Design review of the part built by this model. Coordinates are the model's own, in mm. A direction names the side the tool comes from. Give positions to 0.01 mm unless a question says otherwise; leave off trailing zeros. Loops run counter-clockwise (first coordinate to the right, second up) from the corner with the lowest first, then second, coordinate; pieces in that order, holes last. Notation, with made-up numbers: (8, 37) - (20, 37) arc R22 cw to (20, 55) - close; hole circle Ø1 at (57, -2.75). An arc over 180 degrees is marked (long way). Write each question's results on one line, items separated by ' | '.
from build123d import *

# Parameters (mm, degrees)
SCHIZZO1_R                   = 17.5
ESTRUSIONE_ESTRUSIONE1_DEPTH = 50
TAGLIO_ESTRUSIONE1_REACH     = 145.634
SCHIZZO10_R                  = 16.3
SKETCH1_R                    = 16.3
SKETCH1_R_2                  = 14.8
BOSS_EXTRUDE3_DEPTH          = 15
SKETCH2_R                    = 2.2
BOSS_EXTRUDE4_DEPTH          = 5


# Read off the part's stored shape, not the designer's step: Rivoluzione1
with BuildPart() as part:
    # Schizzo1 → Estrusione-Estrusione1 (new body)
    with BuildSketch(Plane(origin=(0, 0, 0), x_dir=(1, 0, 0), z_dir=(0, 1, 0))):
        with Locations(Location((0, 0, 0), (0, 0, 270))):
            Circle(SCHIZZO1_R)
    extrude(amount=ESTRUSIONE_ESTRUSIONE1_DEPTH)

    # Rivoluzione1 outline → Rivoluzione1 (revolve)
    with BuildSketch(Plane.XY):
        with BuildLine():
            ThreePointArc((2.55, 139.999999998), (1.475612648, 141.087167398), (0, 141.485675179))
            Line((0, 141.485675179), (0, 138.8))
            Line((0, 138.8), (2, 138.8))
            add(Edge.make_bspline(
                [(2, 138.8), (16.3, 113.62789219), (16.3, 50)],
                knots=[0, 0, 0, 1, 1, 1], degree=2))
            Line((16.3, 50), (17.5, 50))
            add(Edge.make_bspline(
                [(17.5, 50), (17.5, 113.62789219), (2.55, 139.999999998)],
                knots=[0.022396988, 0.022396988, 0.022396988, 1.022396988, 1.022396988, 1.022396988], degree=2))
        make_face()
    revolve(axis=Axis((0, 0, 0), (0, 1, 0)))

    # Schizzo10 → Taglio-Estrusione1 (cut, up to next)
    with BuildSketch(Plane(origin=(0, 0, 0), x_dir=(1, 0, 0), z_dir=(0, 1, 0)), mode=Mode.PRIVATE) as taglio_estrusione1_sk1:
        with Locations(Location((0, 0, 0), (0, 0, 270))):
            Circle(SCHIZZO10_R)
    taglio_estrusione1_tool1 = extrude(taglio_estrusione1_sk1.sketch, amount=TAGLIO_ESTRUSIONE1_REACH, mode=Mode.PRIVATE) & part.part
    add(taglio_estrusione1_tool1.solids().sort_by_distance((0, 0, 0))[0], mode=Mode.SUBTRACT)

    # Sketch1 → Boss-Extrude3 (add)
    with BuildSketch(Plane.XZ):
        with Locations(Location((0, 0, 0), (0, 0, 270))):
            Circle(SKETCH1_R)
        with Locations(Location((0, 0, 0), (0, 0, 270))):
            Circle(SKETCH1_R_2, mode=Mode.SUBTRACT)
    extrude(amount=-BOSS_EXTRUDE3_DEPTH)

    # Sketch2 → Boss-Extrude4 (add)
    # profile 1 of 2: a face of its own
    with BuildSketch(Plane.XZ):
        with BuildLine():
            ThreePointArc((8.3, 4.3829214), (3.9170786, 0), (8.3, -4.3829214))
            Line((8.3, -4.3829214), (14.136123938, -4.3829214))
            ThreePointArc((14.136123938, -4.3829214), (14.8, 0), (14.136123938, 4.3829214))
            Line((14.136123938, 4.3829214), (8.3, 4.3829214))
        make_face()
        with Locations(Location((8.3, 0, 0), (0, 0, 270))):
            Circle(SKETCH2_R, mode=Mode.SUBTRACT)
    # profile 2 of 2: a face of its own
    with BuildSketch(Plane.XZ):
        with BuildLine():
            Line((-8.3, 4.3829214), (-14.136123938, 4.3829214))
            ThreePointArc((-14.136123938, 4.3829214), (-14.8, 0), (-14.136123938, -4.3829214))
            Line((-14.136123938, -4.3829214), (-8.3, -4.3829214))
            ThreePointArc((-8.3, -4.3829214), (-3.9170786, 0), (-8.3, 4.3829214))
        make_face()
        with Locations(Location((-8.3, 0, 0), (0, 0, 270))):
            Circle(SKETCH2_R, mode=Mode.SUBTRACT)
    extrude(amount=-BOSS_EXTRUDE4_DEPTH)


solid = part.part
(1) Draft analysis for pull direction Y (two halves, no side actions). For faces 1 (the flat face through (-11, 5, 0)), 2 (the cylindrical face through (-10.448, 2.465, 0.477)), 3 (the flat face through (4.1, 0, 0.2)), state which applies: pulls with the +Y half, pulls with the -Y half, needs draft (parallel to the pull), parting line crosses it, or undercut.
Answers below:
face 1: undercut | face 2: needs draft | face 3: pulls with the -Y half
(2) Insertion check: P1, Ø1, axis at y = 76.5, z = 11, coming from the +X side; P2, Ø2.5, axis at x = -7.5, z = 1.5, coming from the +Y side; P3, Ø4.5, axis at x = -0.5, z = -0.5, coming from the -Y side. Each pin has a flat end and moves straight along its axis. Give the tip position at first contact, or say it passes through.
Answers below:
P1: x = 13.06 | P2: y = 131.99 | P3: y = 137.04
(3) Take a section at A-A on y = 40. Give the boundary of the cut face in (x, z), plus the area to 3 significant figures.
Answers below:
outline: circle Ø35 at (0, 0); hole circle Ø32.6 at (0, 0) | area: 127 mm2
(4) Wall thickness on line 1 along X through (y, z) = (3, 0); line 2 along Z through (x, y) = (0, 30); line 3 along X through (y, z) = (8.25, 0): over which ranges is each line inside the solid? List them lowest first. Write a range as from..to.
Answers below:
line 1: -17.5..-10.5, -6.1..-3.92, 3.92..6.1, 10.5..17.5 | line 2: -17.5..-16.3, 16.3..17.5 | line 3: -17.5..-14.8, 14.8..17.5
(5) Tool access review of faces 4 (the flat face through (-11, 2, 4.383)), 5 (the cylindrical face through (-5.67, 7.4, -13.67)), 6 (the cylindrical face through (-10.648, 24.65, -13.887)): name each direction out of +Z, -Z, +X, -X, +Y, -Y from which nothing blocks a thin tool from reaching the whole face with its end or side.
Answers below:
face 4: -Y | face 5: none | face 6: +Y, -Y
